CAD build for the part. Positions are in the model's coordinates, mm. Face numbers are marked on the shaded views. A direction names the side the tool comes from. Round coordinates to 2 decimals unless told otherwise and drop trailing zeros. Order: outer loops, then holes, each group sorted by start corner. A loop starts at its lowest first (then second) coordinate and runs counter-clockwise, first axis right, second up. Notation, with made-up numbers: (-2.5, 26) - (28.5, 26) arc R23 ccw to (28.5, 41) - close; hole circle Ø2 at (63, 64.25). An arc over 180 degrees is marked (long way). Use one line per item in the form item = value. Start each with the question number.
Autodesk Inventor part; units mm, degrees
ref_plane "YZ Plane" through (0, 0, 0) normal (1, 0, 0) x (0, 1, 0)
ref_plane "XZ Plane" through (0, 0, 0) normal (0, 1, 0) x (-1, 0, 0)
ref_plane "XY Plane" through (0, 0, 0) normal (0, 0, 1) x (1, 0, 0)
sketch "Sketch1" plane through (0, 0, 0) normal (0, 1, 0) x (-1, 0, 0)
  line L0 (-59.7535, -47.0027) -> (59.7535, -47.0027)
  line L1 (59.7535, -47.0027) -> (59.7535, 47.0027)
  line L2 (59.7535, 47.0027) -> (-59.7535, 47.0027)
  line L3 (-59.7535, 47.0027) -> (-59.7535, -47.0027)
  line L4 (-59.7535, -47.0027) -> (59.7535, 47.0027) construction
  line L5 (59.7535, -47.0027) -> (-59.7535, 47.0027) construction
  point P0 (0, 0)
  dimension "d0" = 119.507
  dimension "d1" = 94.0054
extrude "Extrusion1" add sketch "Sketch1" along normal mid plane 2.2606
sketch "Sketch2" plane through (0, 1.1303, 0) normal (0, 1, 0) x (1, 0, 0)
  line L0 (-59.7535, 47.0027) -> (-59.7535, -47.0027)
  line L1 (59.7535, -47.0027) -> (59.7535, 47.0027)
  line L2 (-59.7535, -47.0027) -> (59.7535, -47.0027)
  line L3 (59.7535, -47.0027) -> (59.7535, 47.0027)
  line L4 (59.7535, 47.0027) -> (-59.7535, 47.0027)
  line L5 (-59.7535, 47.0027) -> (-59.7535, -47.0027)
  line L6 (57.4929, -44.7421) -> (-57.4929, 44.7421) construction
  line L7 (-57.4929, -44.7421) -> (57.4929, 44.7421) construction
  line L8 (-59.7535, -47.0027) -> (59.7535, -47.0027)
  line L9 (-59.7535, -47.0027) -> (-50.7619, -47.0027)
  line L10 (-59.7535, -38.0111) -> (-59.7535, -47.0027)
  line L11 (-59.7535, 47.0027) -> (-50.7619, 47.0027)
  line L12 (-59.7535, 38.0111) -> (-59.7535, 47.0027)
  line L13 (59.7535, 47.0027) -> (-59.7535, 47.0027)
  line L14 (59.7535, 47.0027) -> (50.7619, 47.0027)
  line L15 (59.7535, 38.0111) -> (59.7535, 47.0027)
  line L16 (59.7535, -47.0027) -> (50.7619, -47.0027)
  line L17 (59.7535, -38.0111) -> (59.7535, -47.0027)
  line L18 (-50.7619, -44.7421) -> (-50.7619, -38.0111)
  line L19 (-50.7619, -38.0111) -> (-57.4929, -38.0111)
  line L20 (-57.4929, 38.0111) -> (-50.7619, 38.0111)
  line L21 (-50.7619, 38.0111) -> (-50.7619, 44.7421)
  line L22 (50.7619, 38.0111) -> (57.4929, 38.0111)
  line L23 (50.7619, 44.7421) -> (50.7619, 38.0111)
  line L24 (57.4929, -38.0111) -> (50.7619, -38.0111)
  line L25 (50.7619, -38.0111) -> (50.7619, -44.7421)
  line L26 (-50.7619, -44.7421) -> (50.7619, -44.7421)
  line L27 (57.4929, -38.0111) -> (57.4929, 38.0111)
  line L28 (50.7619, 44.7421) -> (-50.7619, 44.7421)
  line L29 (-57.4929, 38.0111) -> (-57.4929, -38.0111)
  point P0 (0, 0)
  dimension "d4" = 114.9858
  dimension "d5" = 89.4842
  dimension "d6" = 8.9916
  dimension "d7" = 8.9916
  dimension "d10" = 8.9916
  dimension "d11" = 8.9916
extrude "Extrusion2" add sketch "Sketch2" along normal blind 101.6
sketch "Sketch3" plane through (0, 1.1303, 0) normal (0, 1, 0) x (1, 0, 0)
  circle A0 centre (0, -25.4) radius 2.0828
  circle A1 centre (0, 25.4) radius 2.0828
  point P0 (0, 0)
  dimension "d18" = 4.1656
  dimension "d19" = 4.1656
extrude "Extrusion3" cut sketch "Sketch3" against normal through all
sketch "Sketch7" plane through (0, 1.1303, 0) normal (0, 1, 0) x (1, 0, 0)
  line L0 (44.6278, -24.4983) -> (-44.6278, 24.4983) construction
  line L1 (-44.6278, -24.4983) -> (44.6278, 24.4983) construction
  line L2 (44.5008, -22.5044) -> (-44.5008, 22.5044) construction
  line L3 (-44.5008, -22.5044) -> (44.5008, 22.5044) construction
  circle A0 centre (41.3258, -19.3294) radius 1.4224
  circle A1 centre (41.3258, 19.3294) radius 1.4224
  circle A2 centre (-41.4528, 20.963) radius 1.4224
  circle A3 centre (-41.4528, -20.963) radius 1.4224
  line L4 (32.9946, -9.9949) -> (-32.9946, 9.9949) construction
  line L5 (-32.9946, -9.9949) -> (32.9946, 9.9949) construction
  circle A4 centre (-32.9946, -9.9949) radius 1.4986
  circle A5 centre (-32.9946, 9.9949) radius 1.4986
  circle A6 centre (32.9946, 9.9949) radius 1.4986
  circle A7 centre (32.9946, -9.9949) radius 1.4986
  point P0 (0, 0)
  point P1 (0, 0)
  dimension "d57" = 2.8448
  dimension "d58" = 2.8448
  dimension "d59" = 2.8448
  dimension "d60" = 2.8448
  dimension "d61" = 65.9892
  dimension "d62" = 19.9898
  dimension "d63" = 2.9972
  dimension "d64" = 2.9972
  dimension "d65" = 2.9972
  dimension "d66" = 2.9972
extrude "Extrusion6" cut sketch "Sketch7" against normal through all
sketch "Sketch8" plane through (-50.7619, 1.1303, -44.7421) normal (0, 0, 1) x (1, 0, 0)
  circle A0 centre (55.4736, 19.05) radius 3.175
  circle A1 centre (83.2549, 19.05) radius 3.175
  point P0 (50.7619, -1.1303)
  dimension "d71" = 6.35
  dimension "d72" = 6.35
extrude "Extrusion7" cut sketch "Sketch8" against normal through all
sketch "Sketch9" plane through (50.7619, 1.1303, 44.7421) normal (0, 0, -1) x (-1, 0, 0)
  line L0 (101.5238, 0) -> (101.5238, 101.6)
  circle A0 centre (18.269, 19.05) radius 3.175
  circle A1 centre (46.0502, 19.05) radius 3.175
  point P0 (50.7619, -1.1303)
  dimension "d79" = 6.35
  dimension "d80" = 6.35
extrude "Extrusion8" cut sketch "Sketch9" against normal through all
properties part number "546-1590BBS-PE4312"
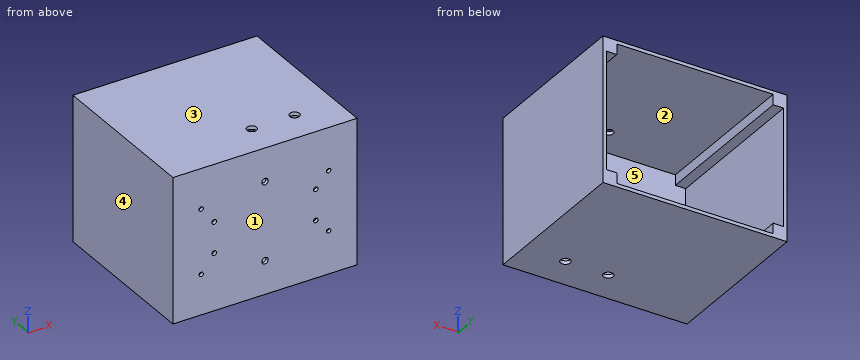
(1) Mould opens along Z. For the marked faces 3, 4 and 5 say: pulls with the +Z half, pulls with the -Z half, needs draft (parallel to the pull), parting line crosses it, or undercut.
(2) Flat gauge pins, fed straight in: P1, Ø2.5, axis at x = 32.99, z = 9.99, coming from the -Y side; P2, Ø5.5, axis at x = 0, z = 25.4, coming from the +Y side. Where does each tip first touch, or does it go through?
(3) Which spindle directions (+Z, -Z, +X, -X, +Y, -Y) get a long thin tool onto all of the face, cutting with end or side? Do the marked faces 1 and 2. Say none if no direction does.
(4) Slice it at D-D (z = 13.5). Give the cut face in (x, y), and give its area (3 significant figures).
(5) Slice it at A-A (z = 25.4). Give the cut face in (x, y).
(6) Slice it at C-C (y = 6.5). Give the cut face in (x, z).
(7) Wall check: line 1 (Z direction, x = 0, y = 0); line 2 (X direction, y = 29, z = -1); line 3 (Z direction, x = -18, y = 73). Give the ranges that are in metal, low to high. Write a range as [from, to].
(8) Slice it at B-B (x = 0). Give the cut face in (y, z).
Results list:
q1.face_3 = pulls with the +Z half
q1.face_4 = needs draft
q1.face_5 = undercut
q2.P1 = through
q2.P2 = 1.13
q3.face_1 = +Z, -Z, +X, -X, -Y
q3.face_2 = +Y
q4.outline = (-59.75, -1.13) - (59.75, -1.13) - (59.75, 102.73) - (57.49, 102.73) - (57.49, 1.13) - (-57.49, 1.13) - (-57.49, 102.73) - (-59.75, 102.73) - close
q4.area = 730 mm²
q5.outline = (-59.75, -1.13) - (-2.08, -1.13) - (-2.08, 1.13) - (-57.49, 1.13) - (-57.49, 102.73) - (-59.75, 102.73) - close; (2.08, -1.13) - (59.75, -1.13) - (59.75, 102.73) - (57.49, 102.73) - (57.49, 1.13) - (2.08, 1.13) - close
q6.outline = (-59.75, -47) - (59.75, -47) - (59.75, 47) - (-59.75, 47) - close; hole (-57.49, -38.01) - (-50.76, -38.01) - (-50.76, -44.74) - (50.76, -44.74) - (50.76, -38.01) - (57.49, -38.01) - (57.49, 38.01) - (50.76, 38.01) - (50.76, 44.74) - (-50.76, 44.74) - (-50.76, 38.01) - (-57.49, 38.01) - close
q7.line_1 = [-47, -27.48], [-23.32, 23.32], [27.48, 47]
q7.line_2 = [-59.75, -57.49], [57.49, 59.75]
q7.line_3 = [-47, -44.74], [44.74, 47]
q8.outline = (-1.13, -47) - (102.73, -47) - (102.73, -44.74) - (1.13, -44.74) - (1.13, -27.48) - (-1.13, -27.48) - close; (-1.13, -23.32) - (1.13, -23.32) - (1.13, 23.32) - (-1.13, 23.32) - close; (-1.13, 27.48) - (1.13, 27.48) - (1.13, 44.74) - (102.73, 44.74) - (102.73, 47) - (-1.13, 47) - close
